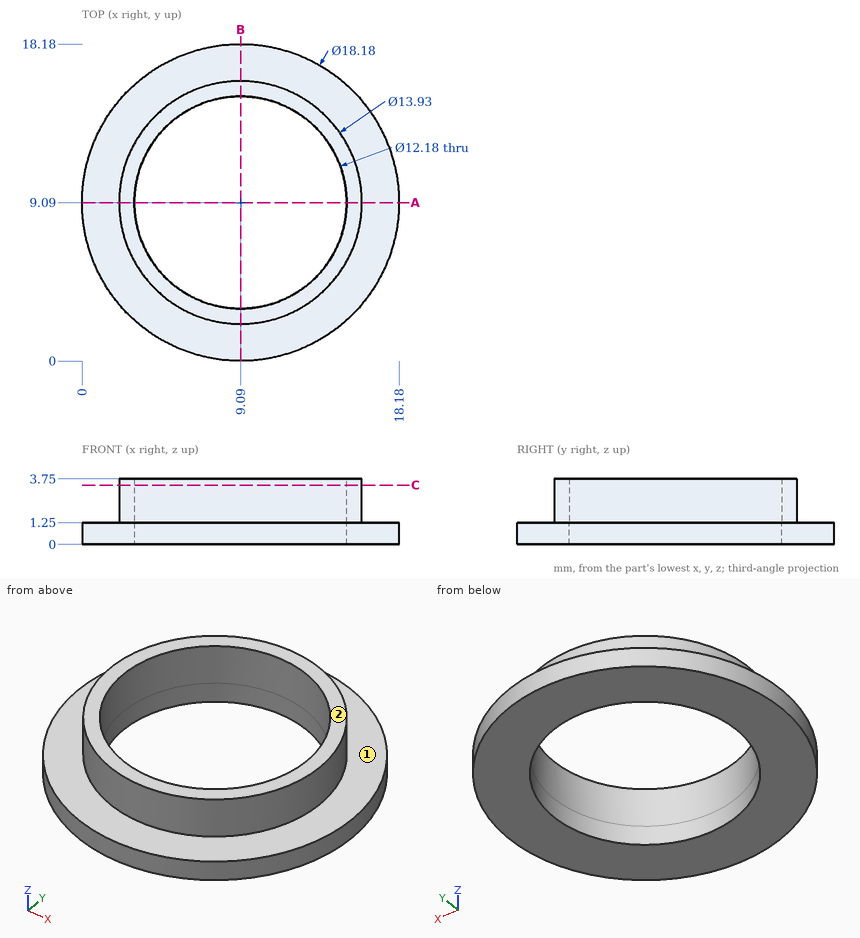
For this review, use the dimensioned drawing (mm, ordinates from the lowest corner) and the shaded views. A direction names the side the tool comes from. Round coordinates to 2 decimals unless told otherwise and drop trailing zeros. Write each loop counter-clockwise with the first axis right and the second up, starting at its lowest first coordinate (ties: lowest second). Pieces come first, ordered by that corner, then holes. Notation, with made-up numbers: M -38.75,70 L -32.75,70 A21 cw -32.75,86 Z; hole C 56,42.25 d2. An arc over 180 degrees is marked long. Write item = value, one per line. Start each with the question number.
(1) For the marked faces 1 and 2, list the 3-axis set-ups (+Z, -Z, +X, -X, +Y, -Y) from which the entire face can be reached by the end or side of a thin tool; tool diameter is ignored.
(2) We need section A-A (y = 9.09). Give the boundary of the cut face in (x, z) (3 decimals).
(3) Clearance check with flat-ended pins moving along their axes: pin 1 Ø1 at (x, z) = (4.5, 2) entering from -Y; pin 2 Ø1.5 at (x, y) = (14.5, 2.5) entering from +Z. State where each tip first meets the part, or that it passes through.
(4) We need section C-C (z = 3.4). Give the boundary of the cut face in (x, y) (3 decimals).
(5) For line 1 along Y through (x, z) = (9.09, 2.65) (3 decimals); line 2 along Z through (x, y) = (14.5, 14); line 3 along Y through (x, z) = (9.09, 0.3), list the stretches that pass through material, from the lowest coordinate up.
Results found:
q1.face_1 = +Z
q1.face_2 = +Z, +X, -X, +Y, -Y
q2.outline = M 0,0 L 3,0 L 3,3.75 L 2.125,3.75 L 2.125,1.25 L 0,1.25 Z; M 15.18,0 L 18.18,0 L 18.18,1.25 L 16.055,1.25 L 16.055,3.75 L 15.18,3.75 Z
q3.pin_1 = 3.45
q3.pin_2 = 1.25
q4.outline = C 9.09,9.09 d13.93; hole C 9.09,9.09 d12.18
q5.line_1 = 2.125 to 3, 15.18 to 16.055
q5.line_2 = 0 to 1.25
q5.line_3 = 0 to 3, 15.18 to 18.18
